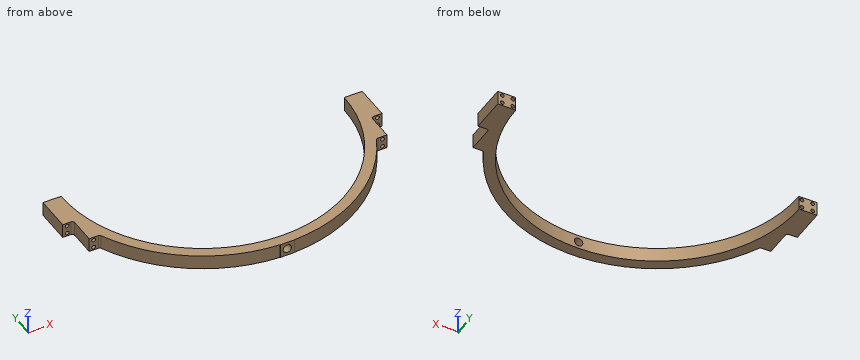
```python
from build123d import *

# Parameters (mm, degrees)
F1_DEPTH = 50.8
F4_D     = 13.49248
F5_D     = 13.49248
F8_D     = 30.1625


with BuildPart() as f1:
    # F0 (on Top) → F1 (new body)
    with BuildSketch(Plane.XY):
        with BuildLine():
            ThreePointArc((0, -508), (-359.2102448428, -359.2102448428), (-508, 0))
            Line((-508, 0), (-546.1, 0))
            Line((-546.1, 0), (-572.4023011247, 0))
            Line((-572.4023011247, 0), (-572.4023011247, -127))
            Line((-572.4023011247, -127), (-542.5175210867, -127))
            ThreePointArc((-542.5175210867, -127), (-536.5306836727, -129.4798292526), (-534.0508544201, -135.4666666667))
            Line((-534.0508544201, -135.4666666667), (-534.0508544201, -228.6))
            Line((-534.0508544201, -228.6), (-501.3417829518, -228.6))
            ThreePointArc((-501.3417829518, -228.6), (-496.8118429706, -229.9137589914), (-493.6877099297, -233.4473282443))
            ThreePointArc((-493.6877099297, -233.4473282443), (-303.0926410641, -454.2687100525), (-26.02025103, -545.47974897))
            Line((-26.02025103, -545.47974897), (-25.4, -546.1))
            Line((-25.4, -546.1), (0, -546.1))
            Line((0, -546.1), (0, -508))
        make_face()
    extrude(amount=F1_DEPTH)

    # F4 (through all)
    with Locations(Plane.XZ.offset(127)):
        with Locations((-556.5273011247, 11.1125), (-556.5273011247, 39.6875)):
            Hole(F4_D / 2)

    # F5 (through all)
    with Locations(Plane.XZ.offset(228.6)):
        with Locations((-518.1758544201, 39.6875), (-518.1758544201, 11.1125)):
            Hole(F5_D / 2)

    # F6: F1 across plane


with BuildPart() as f1_1:
    add(f1.part)
    add(f1.part.mirror(Plane.YZ))

    # F8 (through all)
    with Locations(Plane.XZ.offset(546.1)):
        with Locations((0, 25.4)):
            Hole(F8_D / 2)


solid = f1_1.part
```
For this review, take the finished solid that the model builds, in its own axes (mm). Round coordinates to 2 decimals unless told otherwise and drop trailing zeros. Write each loop counter-clockwise with the first axis right and the second up, starting at its lowest first coordinate (ties: lowest second). Pieces come first, ordered by that corner, then holes. Notation, with made-up numbers: (0.25, 39.25) - (28.25, 39.25) arc R18 cw to (28.25, 46.25) - close; hole circle Ø11 at (-15, -21.5). An arc over 180 degrees is marked (long way). Answer as CSV lines item,"result". Start each with the question number.
(1) For line 1 (Z direction, x = 0, y = -526); line 2 (X direction, y = -40.5, z = 8.5); line 3 (X direction, y = -129, z = 34.5), list the stretches that pass through material, from the lowest coordinate up.
(2) Add section B-B, the plane y = -146. State the section outline as (x, z) points, plus the area to 3 significant figures.
(3) Add section D-D, the plane x = -217. State the section outline as (y, z) points, plus the area to 3 significant figures.
(4) Add section A-A, the plane x = 0. State the section outline as (y, z) points, plus the area to 3 significant figures.
(5) For pin 1 (12 mm diameter, centred on x = -556.53, z = 39.69, fed in from +Y); pin 2 (16.5 mm diameter, centred on x = 518, z = 34.5, fed in from -Y); pin 3 (15 mm diameter, centred on x = -556.5, z = 28.5, fed in from -Y); pin 4 (5 mm diameter, centred on x = 160.5, z = 23, fed in from +Y), all flat-tipped, find the tip position at first contact; note any pin that passes through.
(6) Add section C-C, the plane y = -209. State the section outline as (x, z) points.
From the geometry:
1,line 1,"z = 0 to 10.32, 40.48 to 50.8"
1,line 2,"x = -572.4 to -562.75, -550.31 to -524.4, -511.96 to -506.38, 506.38 to 511.96, 524.4 to 550.31, 562.75 to 572.4"
1,line 3,"x = -537.05 to -522.49, -513.86 to -491.35, 491.35 to 513.86, 522.49 to 537.05"
2,outline,"(-534.05, 0) - (-486.57, 0) - (-486.57, 50.8) - (-534.05, 50.8) - close; (486.57, 0) - (534.05, 0) - (534.05, 50.8) - (486.57, 50.8) - close; hole circle Ø13.49 at (-518.18, 11.11); hole circle Ø13.49 at (-518.18, 39.69); hole circle Ø13.49 at (518.18, 11.11); hole circle Ø13.49 at (518.18, 39.69)"
2,area,"4,250 mm²"
3,outline,"(-501.13, 0) - (-459.32, 0) - (-459.32, 50.8) - (-501.13, 50.8) - close"
3,area,"2,120 mm²"
4,outline,"(-546.1, 0) - (-508, 0) - (-508, 10.32) - (-546.1, 10.32) - close; (-546.1, 40.48) - (-508, 40.48) - (-508, 50.8) - (-546.1, 50.8) - close"
4,area,"786 mm²"
5,pin 1,"passes through"
5,pin 2,"stops at y = -228.6"
5,pin 3,"stops at y = -127"
5,pin 4,"stops at y = -481.14"
6,outline,"(-534.05, 0) - (-463.02, 0) - (-463.02, 50.8) - (-534.05, 50.8) - close; (463.02, 0) - (534.05, 0) - (534.05, 50.8) - (463.02, 50.8) - close; hole circle Ø13.49 at (-518.18, 11.11); hole circle Ø13.49 at (-518.18, 39.69); hole circle Ø13.49 at (518.18, 11.11); hole circle Ø13.49 at (518.18, 39.69)"
